Design review of the part built by this model. Coordinates are the model's own, in mm. A direction names the side the tool comes from. Round coordinates to 2 decimals unless told otherwise and drop trailing zeros. Loops run counter-clockwise (first coordinate to the right, second up) from the corner with the lowest first, then second, coordinate; pieces in that order, holes last. Notation, with made-up numbers: M -32,69 L -16,69 A29 ccw -16,100 Z; hole C -37.75,-33 d2. An arc over 180 degrees is marked long. One line per item, written item: value. Start each with the question number.
Item 1: Clearance check with flat-ended pins moving along their axes: pin 1 (4 mm diameter, centred on x = 750.5, y = -2, fed in from +Z); pin 2 (8 mm diameter, centred on x = 772.5, y = -22, fed in from -Z); pin 3 (2 mm diameter, centred on x = 769, y = -32.5, fed in from -Z); pin 4 (1 mm diameter, centred on x = 739.5, y = -43.5, fed in from -Z). State where each tip first meets the part, or that it passes through.
Item 2: For line 1 along Y through (x, z) = (734.5, 511.5); line 2 along X through (y, z) = (11.5, 495); line 3 along X through (y, z) = (-20, 501.5), list the stretches that pass through material, from the lowest coordinate up.
Item 3: We need section B-B (z = 515). Write out the cut boundary in (x, y).
Item 4: We need section A-A (x = 757.5). Write out the cut boundary in (y, z).
Item 5: For faces 1 (the cylindrical face through (766.1, -36.34, 501.51)), 2 (the flat face through (757, -60, 515)), list the 3-axis set-ups (+Z, -Z, +X, -X, +Y, -Y) from which the entire face can be reached by the end or side of a thin tool; tool diameter is ignored.
Item 6: We need section D-D (z = 495). Write out the cut boundary in (x, y), then the cut area to 3 significant figures.
Item 7: We need section C-C (y = -32). Write out the cut boundary in (x, z), then the cut area to 3 significant figures.
from build123d import *

# Parameters (mm, degrees)
EXTRUDE_START          = -60
EXTRUDE_SKETCH_1_R     = 16
EXTRUDE_1_DEPTH        = 48
EXTRUDE_ROTATE_1_ANGLE = 90
EXTRUDE_START_2        = -12
EXTRUDE_SKETCH_2_R     = 26
EXTRUDE_2_DEPTH        = 26
EXTRUDE_ROTATE_2_ANGLE = 90


with BuildPart() as part:
    # Extrude sketch 1 → Extrude 1 (new body)
    with BuildSketch(Plane.XY.offset(EXTRUDE_START)):
        Circle(EXTRUDE_SKETCH_1_R)
    extrude(amount=EXTRUDE_1_DEPTH)


with BuildPart() as part_1:
    # Extrude rotate 1: moved
    add(part.part.rotate(Axis((0, 0, 0), (-1, 0, 0)), EXTRUDE_ROTATE_1_ANGLE))


with BuildPart() as part_2:
    # Extrude place 1: moved
    add(part_1.part.moved(Location((757.5, 0, 515))))


with BuildPart() as body_2:
    # Extrude sketch 2 → Extrude 2 (new body)
    with BuildSketch(Plane.XY.offset(EXTRUDE_START_2)):
        Circle(EXTRUDE_SKETCH_2_R)
    extrude(amount=EXTRUDE_2_DEPTH)


with BuildPart() as body_2_1:
    # Extrude rotate 2: moved
    add(body_2.part.rotate(Axis((0, 0, 0), (-1, 0, 0)), EXTRUDE_ROTATE_2_ANGLE))


with BuildPart() as body_2_2:
    # Extrude place 2: moved
    add(body_2_1.part.moved(Location((757.5, 0, 515))))


with BuildPart() as part_3:
    add(part_2.part)

    # Combine (weld / assembly of features): union body 2
    add(body_2_2.part)


solid = part_3.part
A:
1. pin 1: z = 540.51
1. pin 2: z = 503.38
1. pin 3: z = 502.93
1. pin 4: through
2. line 1: -12 to 14
2. line 2: 740.89 to 774.11
2. line 3: 748.91 to 766.09
3. outline: M 731.5,-12 L 741.5,-12 L 741.5,-60 L 773.5,-60 L 773.5,-12 L 783.5,-12 L 783.5,14 L 731.5,14 Z
4. outline: M -60,499 L -12,499 L -12,489 L 14,489 L 14,541 L -12,541 L -12,531 L -60,531 Z
5. face 1: -Y
5. face 2: +Z, -Z, +X, -X, -Y
6. outline: M 740.89,-12 L 774.11,-12 L 774.11,14 L 740.89,14 Z
6. area: 864 mm2
7. outline: C 757.5,515 d32
7. area: 804 mm2
